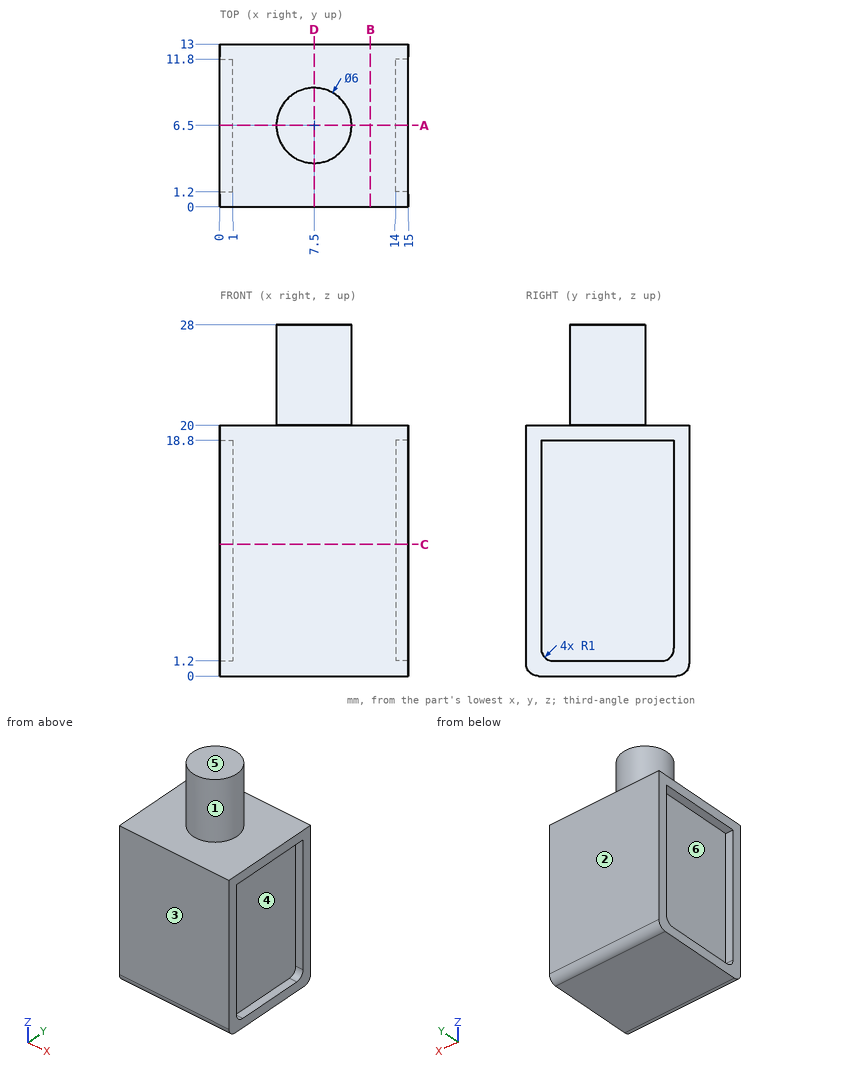
Answer from the drawing. Dimensions are ordinates in mm from the lowest x, y and z of the part. A direction names the side the tool comes from. Round coordinates to 2 decimals unless told otherwise and drop trailing zeros. Write each loop counter-clockwise with the first axis right and the second up, starting at its lowest first coordinate (ties: lowest second). Pieces come first, ordered by that corner, then holes. Notation, with made-up numbers: M 46.5,63 L 94.5,63 A12 ccw 94.5,72 Z; hole C -22,-17 d7. An arc over 180 degrees is marked long. Write each question's results on one line, items separated by ' | '. Start each with the question number.
Item 1: A cutting plane is placed at B-B on x = 12. Write down the section's boundary in (y, z).
Item 2: A cutting plane is placed at A-A on y = 6.5. Write down the section's boundary in (x, z).
Item 3: Straight lines are drawn through the part: L1, parallel to Z at x = 11.5, y = 9.25; L2, parallel to X at y = 6.25, z = 9.75; L3, parallel to X at y = 7, z = 26.75. For each, find the intervals that lie inside material, in ascending order. Write a range as [from, to].
Item 4: Flat-ended cylindrical pins translate along their axes: pin 1 Ø1 at (y, z) = (5, 9) entering from +X; pin 2 Ø1.5 at (x, z) = (8.5, 22) entering from -Y; pin 3 Ø1.1 at (x, y) = (0.5, 7.5) entering from +Z. Find the tip coordinate at first contact, or state that the pin passes through.
Item 5: For the marked faces 1 and 2, determine the directions among +Z, -Z, +X, -X, +Y, -Y from which every point of the face is accessible in a straight line to the end or side of a thin tool.
Item 6: A cutting plane is placed at C-C on z = 10.5. Write down the section's boundary in (x, y), and give its area (3 significant figures).
Item 7: For a pull along Y with two mould halves and no side action, classify the marked faces 3, 4, 5 and 6 as pulls with the +Y half, pulls with the -Y half, needs draft (parallel to the pull), parting line crosses it, or undercut.
Item 8: A cutting plane is placed at D-D on x = 7.5. Write down the section's boundary in (y, z), and give its area (3 significant figures).
Check sheet entries:
1) outline: M 0,1 A1 ccw 1,0 L 12,0 A1 ccw 13,1 L 13,20 L 0,20 Z
2) outline: M 0,0 L 15,0 L 15,1.2 L 14,1.2 L 14,18.8 L 15,18.8 L 15,20 L 10.5,20 L 10.5,28 L 4.5,28 L 4.5,20 L 0,20 L 0,18.8 L 1,18.8 L 1,1.2 L 0,1.2 Z
3) L1: [0, 20] | L2: [1, 14] | L3: [4.54, 10.46]
4) pin 1: x = 14 | pin 2: y = 3.51 | pin 3: z = 20
5) face 1: +Z | face 2: +Z, -Z, +X, -X, +Y
6) outline: M 0,0 L 15,0 L 15,1.2 L 14,1.2 L 14,11.8 L 15,11.8 L 15,13 L 0,13 L 0,11.8 L 1,11.8 L 1,1.2 L 0,1.2 Z | area: 174 mm²
7) face 3: pulls with the -Y half | face 4: undercut | face 5: needs draft | face 6: undercut
8) outline: M 0,1 A1 ccw 1,0 L 12,0 A1 ccw 13,1 L 13,20 L 9.5,20 L 9.5,28 L 3.5,28 L 3.5,20 L 0,20 Z | area: 308 mm²
